CAD build for the part. Positions are in the model's coordinates, mm. Face numbers are marked on the shaded views. A direction names the side the tool comes from. Round coordinates to 2 decimals unless told otherwise and drop trailing zeros. Loops run counter-clockwise (first coordinate to the right, second up) from the corner with the lowest first, then second, coordinate; pieces in that order, holes last. Notation, with made-up numbers: M 21.25,18 L 32.25,18 A24 cw 32.25,43 Z; hole C 20,-38 d11. An arc over 180 degrees is marked long. Use one line per item in the form item = value.
from build123d import *

# Parameters (mm, degrees)
SKETCH1_W                = 4
SKETCH1_H                = 40
BOSS_EXTRUDE2_DEPTH      = 20
BOSS_EXTRUDE2_DEPTH_BACK = 4
SKETCH3_R                = 1.5
CUT_EXTRUDE1_DEPTH       = 29.565713714
SKETCH4_W                = 3
SKETCH4_H                = 40
BOSS_EXTRUDE3_DEPTH      = 10
SKETCH5_R                = 1.5
CUT_EXTRUDE2_DEPTH       = 39.288379438
SKETCH8_W                = 14
SKETCH8_H                = 40
SKETCH8_R                = 1.5
BOSS_EXTRUDE4_DEPTH      = 2
BOSS_EXTRUDE5_DEPTH      = 40
FILLET3_R                = 1


with BuildPart() as part:
    # Sketch1 → Boss-Extrude2 (new, two sides)
    with BuildSketch(Plane.XY) as boss_extrude2_sk:
        with Locations((13, 0)):
            Rectangle(SKETCH1_W, SKETCH1_H)
    extrude(amount=BOSS_EXTRUDE2_DEPTH)
    extrude(boss_extrude2_sk.sketch, amount=-BOSS_EXTRUDE2_DEPTH_BACK)

    # Sketch3 → Cut-Extrude1 (cut, through all)
    with BuildSketch(Plane(origin=(15, 0, 0), x_dir=(0, 0, -1), z_dir=(1, 0, 0))):
        with Locations((-7.5, -16)):
            Circle(SKETCH3_R)
        with Locations((-7.5, 11.5)):
            Circle(SKETCH3_R)
        with Locations((-0.5, 11.5)):
            Circle(SKETCH3_R)
        with Locations((-0.5, -16)):
            Circle(SKETCH3_R)
    extrude(amount=-CUT_EXTRUDE1_DEPTH, mode=Mode.SUBTRACT)

    # Sketch4 → Boss-Extrude3 (add)
    with BuildSketch(Plane(origin=(15, 0, 0), x_dir=(0, 0, -1), z_dir=(1, 0, 0))):
        with Locations((-18.5, 0)):
            Rectangle(SKETCH4_W, SKETCH4_H)
    extrude(amount=BOSS_EXTRUDE3_DEPTH)

    # Sketch5 → Cut-Extrude2 (cut, through all)
    with BuildSketch(Plane(origin=(0, 0, 17), x_dir=(-1, 0, 0), z_dir=(0, 0, -1))):
        with Locations(Location((-19.5, -10, 0), (0, 0, 90))):
            Circle(SKETCH5_R)
        with Locations(Location((-19.5, 10, 0), (0, 0, 90))):
            Circle(SKETCH5_R)
    extrude(amount=-CUT_EXTRUDE2_DEPTH, mode=Mode.SUBTRACT)

    # Sketch8 → Boss-Extrude4 (add)
    with BuildSketch(Plane.XY.offset(20)):
        with Locations((18, 0)):
            Rectangle(SKETCH8_W, SKETCH8_H)
        with Locations(Location((19.5, 10, 0), (0, 0, 90))):
            Circle(SKETCH8_R, mode=Mode.SUBTRACT)
        with Locations(Location((19.5, -10, 0), (0, 0, 90))):
            Circle(SKETCH8_R, mode=Mode.SUBTRACT)
    extrude(amount=BOSS_EXTRUDE4_DEPTH)

    # Sketch9 → Boss-Extrude5 (add)
    with BuildSketch(Plane.XZ.offset(20)):
        Polygon((17, 17), (15, 17), (15, 15.5), align=None)
    extrude(amount=-BOSS_EXTRUDE5_DEPTH)

    # Fillet3
    fillet3_edges = [part.edges().sort_by_distance(p)[0] for p in [
        (15, 0, 15.5),
        (17, 0, 17),
    ]]
    fillet(fillet3_edges, radius=FILLET3_R)


solid = part.part
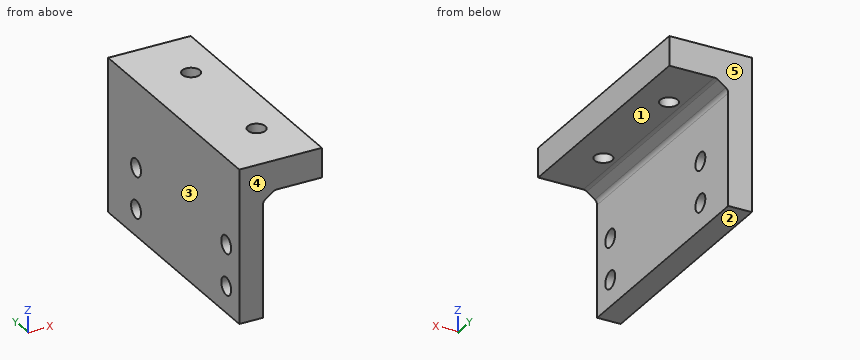
1. Cut at C-C on z = 18.5. Write the cut outline in (x, y).
Completed:
outline = M 11,-20 L 25,-20 L 25,20 L 11,20 Z; hole C 19.5,-10 d3; hole C 19.5,10 d3
2. Tool access for the marked faces 1 and 2: list every direction of +Z, -Z, +X, -X, +Y, -Y with a clear straight run to the whole face (end or side of a thin tool).
Completed:
face_1 = -Z, +X, +Y, -Y
face_2 = -Z, +X, -X, +Y, -Y
3. Cut at A-A on y = -10. Write the cut outline in (x, z), and give its area (3 significant figures).
Completed:
outline = M 11,-4 L 15,-4 L 15,15 A1 cw 15.4,15.8 L 16.73,16.8 A1 cw 17.33,17 L 18,17 L 18,22 L 11,22 Z; M 21,17 L 25,17 L 25,22 L 21,22 Z
area = 141 mm2
4. Cut at B-B on x = 19.5. Write the cut outline in (y, z), and give its area (3 significant figures).
Completed:
outline = M -20,17 L -11.5,17 L -11.5,22 L -20,22 Z; M -8.5,17 L 8.5,17 L 8.5,22 L -8.5,22 Z; M 11.5,17 L 20,17 L 20,22 L 11.5,22 Z
area = 170 mm2
5. Drop flat-ended pins along their axis: P1, Ø10, axis at y = 15, z = -1, coming from the +X side; P2, Ø6, axis at x = 21.5, y = 9.5, coming from the -Z side. Give the stop position or say it passes through.
Completed:
P1 = 15
P2 = 17
6. Pull direction Y, two halves, no side cores. Call the marked faces 3, 4 and 5: +Y half, -Y half, draft (parallel to the pull), parting line (faces both ways), or undercut.
Completed:
face_3 = draft
face_4 = -Y half
face_5 = +Y half
7. Cut at D-D on y = -16. Write the cut outline in (x, z), and give its area (3 significant figures).
Completed:
outline = M 11,-4 L 15,-4 L 15,-1 L 11,-1 Z; M 11,2 L 15,2 L 15,6 L 11,6 Z; M 11,9 L 15,9 L 15,15 A1 cw 15.4,15.8 L 16.73,16.8 A1 cw 17.33,17 L 25,17 L 25,22 L 11,22 Z
area = 132 mm2
8. Probe line 1 along Y through (x, z) = (14.05, 7.5); line 2 along Y through (x, z) = (19.5, 20); line 3 along Z through (x, y) = (24.25, -8.5). List the from-to ranges inside material, lowest first. Write a range as from..to.
Completed:
line_1 = -20..-17.5, -14.5..10, 13..20
line_2 = -20..-11.5, -8.5..8.5, 11.5..20
line_3 = 17..22
